Could you check a few things on this model? Use its own coordinates, in mm. A direction names the side the tool comes from. Round coordinates to 2 decimals unless told otherwise and drop trailing zeros. Order: outer loops, then holes, each group sorted by start corner. A loop starts at its lowest first (then second) coordinate and runs counter-clockwise, first axis right, second up. Notation, with made-up numbers: (64.5, 39.25) - (118.5, 39.25) arc R37 cw to (118.5, 78.25) - close; hole circle Ø6 at (11, 22.5). An arc over 180 degrees is marked (long way). Use one line per item in the form item = value.
from build123d import *

# Parameters (mm, degrees)
SKETCH1_W                                           = 80
SKETCH1_H                                           = 80
SKETCH1_R                                           = 11
BOSS_EXTRUDE1_DEPTH                                 = 10
CSK_FOR_M3_COUNTERSUNK_FLAT_HEAD_SCREW1_D           = 3.2
CSK_FOR_M3_COUNTERSUNK_FLAT_HEAD_SCREW1_CSINK_D     = 6.3
CSK_FOR_M3_COUNTERSUNK_FLAT_HEAD_SCREW1_CSINK_ANGLE = 90
SKETCH5_W                                           = 10
SKETCH5_H                                           = 80
BOSS_EXTRUDE2_DEPTH                                 = 70
BOSS_EXTRUDE3_DEPTH                                 = 10
CSK_FOR_M5_COUNTERSUNK_FLAT_HEAD_SCREW1_D           = 5.3
CSK_FOR_M5_COUNTERSUNK_FLAT_HEAD_SCREW1_CSINK_D     = 10.4
CSK_FOR_M5_COUNTERSUNK_FLAT_HEAD_SCREW1_CSINK_ANGLE = 90
FILLET1_R                                           = 10


with BuildPart() as part:
    # Sketch1 → Boss-Extrude1 (new body)
    with BuildSketch(Plane(origin=(0, 0, 0), x_dir=(1, 0, 0), z_dir=(0, 1, 0))):
        Rectangle(SKETCH1_W, SKETCH1_H)
        with Locations(Location((0, 0, 0), (0, 0, 270))):
            Circle(SKETCH1_R, mode=Mode.SUBTRACT)
    extrude(amount=BOSS_EXTRUDE1_DEPTH)

    # CSK for M3 Countersunk Flat Head Screw1 (through all)
    with Locations(Plane(origin=(0, 10, 0), x_dir=(1, 0, 0), z_dir=(0, 1, 0))):
        with Locations((-15.5, 15.5), (15.5, 15.5), (15.5, -15.5), (-15.5, -15.5)):
            CounterSinkHole(CSK_FOR_M3_COUNTERSUNK_FLAT_HEAD_SCREW1_D / 2, CSK_FOR_M3_COUNTERSUNK_FLAT_HEAD_SCREW1_CSINK_D / 2, counter_sink_angle=CSK_FOR_M3_COUNTERSUNK_FLAT_HEAD_SCREW1_CSINK_ANGLE)

    # Sketch5 → Boss-Extrude2 (add)
    with BuildSketch(Plane(origin=(0, 0, 0), x_dir=(-1, 0, 0), z_dir=(0, -1, 0))):
        with Locations((-35, 0)):
            Rectangle(SKETCH5_W, SKETCH5_H)
    extrude(amount=BOSS_EXTRUDE2_DEPTH)

    # Sketch6 → Boss-Extrude3 (add)
    with BuildSketch(Plane.XY.offset(40)):
        Polygon((-11.715728753, 0), (-18.786796564, 0), (-15.251262658, -3.535533906), (26.464466094, -45.251262658), (30, -48.786796564), (30, -41.715728753), align=None)
        Polygon((-32.928932188, 0), (-40, 0), (30, -70), (30, -62.928932188), align=None)
    boss_extrude3 = extrude(amount=-BOSS_EXTRUDE3_DEPTH)

    # Mirror1: Boss-Extrude3 across plane
    add(boss_extrude3.mirror(Plane.XY))

    # CSK for M5 Countersunk Flat Head Screw1 (through all)
    with Locations(Plane.ZY.offset(-30)):
        with Locations((15, -20), (15, -50), (-15, -50), (-15, -20)):
            CounterSinkHole(CSK_FOR_M5_COUNTERSUNK_FLAT_HEAD_SCREW1_D / 2, CSK_FOR_M5_COUNTERSUNK_FLAT_HEAD_SCREW1_CSINK_D / 2, counter_sink_angle=CSK_FOR_M5_COUNTERSUNK_FLAT_HEAD_SCREW1_CSINK_ANGLE)

    # Fillet1
    # the kernel refuses this fillet: 10 mm, written as the material it takes off along each edge
    with BuildSketch(Plane(origin=(-40, -25, -40), x_dir=(1, 0, 0), z_dir=(0, 1, 0))) as fillet1_piece_1:
        with BuildLine():
            CenterArc((FILLET1_R, -FILLET1_R), FILLET1_R, 90, 90)
            Line((0, -FILLET1_R), (0, 0))
            Line((0, 0), (FILLET1_R, 0))
        make_face()
    extrude(amount=60, mode=Mode.SUBTRACT)
    with BuildSketch(Plane(origin=(-40, -25, 40), x_dir=(1, 0, 0), z_dir=(0, 1, 0))) as fillet1_piece_2:
        with BuildLine():
            CenterArc((FILLET1_R, FILLET1_R), FILLET1_R, 180, 90)
            Line((0, FILLET1_R), (0, 0))
            Line((0, 0), (FILLET1_R, 0))
        make_face()
    extrude(amount=60, mode=Mode.SUBTRACT)


solid = part.part
Item 1: Imagine slicing it at C-C on z = 8.5. Please give me the cut outline in (x, y), plus the area to 3 significant figures.
Found:
outline = (-40, 0) - (-6.98, 0) - (-6.98, 10) - (-40, 10) - close; (6.98, 0) - (30, 0) - (30, -70) - (40, -70) - (40, 10) - (6.98, 10) - close
area = 1,360 mm2
Item 2: Imagine slicing it at A-A on x = 0. Please give me the cut outline in (y, z).
Found:
outline = (-40, -40) - (-32.93, -40) - (-32.93, -30) - (-40, -30) - close; (-40, 30) - (-32.93, 30) - (-32.93, 40) - (-40, 40) - close; (-18.79, -40) - (-11.72, -40) - (-11.72, -30) - (-18.79, -30) - close; (-18.79, 30) - (-11.72, 30) - (-11.72, 40) - (-18.79, 40) - close; (0, -40) - (10, -40) - (10, -11) - (0, -11) - close; (0, 11) - (10, 11) - (10, 40) - (0, 40) - close
Item 3: Will these pins go through, and if not, where does the flat tip stop? P1, Ø8, axis at y = -59, z = 23, coming from the -X side; P2, Ø6, axis at x = 9, z = -9.5, coming from the -Y side; P3, Ø24.5, axis at x = 11, y = -22, coming from the +Z side; P4, Ø4, axis at x = -15.5, z = -15.5, coming from the +Y side.
Found:
P1 = 30
P2 = 0
P3 = 40
P4 = 8.85
Item 4: I need wall thicknesses on L1, parallel to Z at x = -15.5, y = 6; L2, parallel to Z at x = 38, y = -50; L3, parallel to Y at x = 36, z = -15. Which ranges of each line are inside material? Lowest first, please.
Found:
L1 = -40 to -17.1, -13.9 to 13.9, 17.1 to 40
L2 = -40 to -17.65, -12.35 to 12.35, 17.65 to 40
L3 = -70 to -52.65, -47.35 to -22.65, -17.35 to 10
Item 5: If we mould it in two halves opening along Z, with no side actions, what happens to faces 4 (the face through (10, -24, 40)), 5 (the face through (30, -35, 1)), 6 (the face through (-9, 10, -9))? For each: released by +Z, released by -Z, zero draft, split by the parting line, or undercut.
Found:
face_4 = released by +Z
face_5 = undercut
face_6 = zero draft
Item 6: For faces 1 (the face through (5.265, -24.052, 35.07)), 2 (the face through (7, -22, 30)), 3 (the face through (36.327, -47.766, 13.575)), which set-ups out of +Z, -Z, +X, -X, +Y, -Y let a thin tool reach every point of the face, with its end or its side?
Found:
face_1 = +Z, -Z
face_2 = -X, -Y
face_3 = +X, -X
Item 7: Imagine slicing it at D-D on z = 24.5. Please give me the cut outline in (x, y), plus the area to 3 significant figures.
Found:
outline = (-40, 0) - (30, 0) - (30, -70) - (40, -70) - (40, 10) - (-40, 10) - close
area = 1,500 mm2
Item 8: Imagine slicing it at B-B on y = -13.5. Please give me the cut outline in (x, z).
Found:
outline = (-26.5, -40) - (-19.43, -40) - (-19.43, -30) - (-26.5, -30) - close; (-26.5, 30) - (-19.43, 30) - (-19.43, 40) - (-26.5, 40) - close; (-5.29, -40) - (1.78, -40) - (1.78, -30) - (-5.29, -30) - close; (-5.29, 30) - (1.78, 30) - (1.78, 40) - (-5.29, 40) - close; (30, -40) - (40, -40) - (40, 40) - (30, 40) - close
